Model file for the job. Use its own axes, mm. A direction names the side the tool comes from. Give positions to 0.01 mm unless a question says otherwise; leave off trailing zeros. Loops run counter-clockwise (first coordinate to the right, second up) from the corner with the lowest first, then second, coordinate; pieces in that order, holes last. Notation, with made-up numbers: (-13.75, -19) - (0.25, -19) arc R8 cw to (0.25, -11) - close; hole circle Ø7 at (88, 85). An arc over 180 degrees is marked (long way). Answer as CSV lines item,"result". Start each with the question number.
Item 1: Saw through at C-C on y = -2.75. Give the cut face in (x, z).
Item 2: Saw through at A-A on x = 0. Give the cut face in (y, z), plus the area to 3 significant figures.
Item 3: Drill centre lines: L1, parallel to Z at x = 19, y = 1.25; L2, parallel to Y at x = -2, z = 9.5; L3, parallel to X at y = 4.5, z = 10.5. Where is each one in solid material? Low to high. Write a range as from..to.
Item 4: Saw through at D-D on x = 18.5. Give the cut face in (y, z), plus the area to 3 significant figures.
Item 5: Tool access for faces 1 (the flat face through (-6, -3, 25.4)), 2 (the flat face through (18, 6.35, 6)): list every direction of +Z, -Z, +X, -X, +Y, -Y with a clear straight run to the whole face (end or side of a thin tool).
Item 6: Saw through at B-B on z = 5.5. Give the cut face in (x, y), plus the area to 3 significant figures.
Item 7: Pin check, flat tips, straight feed: pin 1 (14 mm diameter, centred on x = 19, z = 5, fed in from +Y); pin 2 (4 mm diameter, centred on y = 4.5, z = 8, fed in from +X); pin 3 (2 mm diameter, centred on x = 7, z = 14, fed in from +Y); pin 4 (2.5 mm diameter, centred on x = 16.5, y = -1.5, fed in from +Z). Stop position of each tip, or through.
Item 8: Pull direction X, two halves, no side cores. Call faces 3 (the flat face through (18, -6.35, 6)), 4 (the flat face through (25.4, 0, 3)), 5 (the cylindrical face through (-1.38, -6.2, 12.52)): pulls with the +X half, pulls with the -X half, needs draft (parallel to the pull), parting line crosses it, or undercut.
from build123d import *

# Parameters (mm, degrees)
F0_R     = 6.35
F1_DEPTH = 25.4
F0_W     = 6.35
F0_H     = 6.35
F2_DEPTH = 12.7
F3_SIZE  = 6.35


with BuildPart() as f1:
    # F0 (on Top) → F1 (new body)
    with BuildSketch(Plane.XY):
        with BuildLine():
            ThreePointArc((10.9985226281, -6.35), (12.2672579939, -3.2870018728), (12.7, 0))
            ThreePointArc((12.7, 0), (12.2672579939, 3.2870018728), (10.9985226281, 6.35))
            ThreePointArc((10.9985226281, 6.35), (-12.7, 0), (10.9985226281, -6.35))
        make_face()
        Circle(F0_R, mode=Mode.SUBTRACT)
    extrude(amount=F1_DEPTH)

    # F0 (on Top) → F2 (join)
    with BuildSketch(Plane.XY):
        with BuildLine():
            Line((19.05, 0), (12.7, 0))
            ThreePointArc((12.7, 0), (12.2672579939, -3.2870018728), (10.9985226281, -6.35))
            Line((10.9985226281, -6.35), (19.05, -6.35))
            Line((19.05, -6.35), (19.05, 0))
        make_face()
        with BuildLine():
            ThreePointArc((10.9985226281, 6.35), (12.2672579939, 3.2870018728), (12.7, 0))
            Line((12.7, 0), (19.05, 0))
            Line((19.05, 0), (19.05, 6.35))
            Line((19.05, 6.35), (10.9985226281, 6.35))
        make_face()
        with Locations((22.225, 3.175)):
            Rectangle(F0_W, F0_H)
        with Locations((22.225, -3.175)):
            Rectangle(F0_W, F0_H)
    extrude(amount=F2_DEPTH)

    # F3
    f3_edges = [f1.edges().sort_by_distance(p)[0] for p in [
        (25.4, 0, 12.7),
    ]]
    chamfer(f3_edges, length=F3_SIZE)


solid = f1.part
Responses:
1,outline,"(-12.4, 0) - (-5.72, 0) - (-5.72, 25.4) - (-12.4, 25.4) - close; (5.72, 0) - (25.4, 0) - (25.4, 6.35) - (19.05, 12.7) - (12.4, 12.7) - (12.4, 25.4) - (5.72, 25.4) - close"
2,outline,"(-12.7, 0) - (-6.35, 0) - (-6.35, 25.4) - (-12.7, 25.4) - close; (6.35, 0) - (12.7, 0) - (12.7, 25.4) - (6.35, 25.4) - close"
2,area,"323 mm2"
3,L1,"0..12.7"
3,L2,"-12.54..-6.03, 6.03..12.54"
3,L3,"-11.88..-4.48, 4.48..21.25"
4,outline,"(-6.35, 0) - (6.35, 0) - (6.35, 12.7) - (-6.35, 12.7) - close"
4,area,"161 mm2"
5,face 1,"+Z, +X, -X, +Y, -Y"
5,face 2,"+Z, -Z, +X, +Y"
6,outline,"(11, -6.35) - (25.4, -6.35) - (25.4, 6.35) - (11, 6.35) arc R12.7 ccw (long way) to start; hole circle Ø12.7 at (0, 0)"
6,area,"548 mm2"
7,pin 1,"y = 6.35"
7,pin 2,"x = 25.4"
7,pin 3,"y = 11.19"
7,pin 4,"z = 12.7"
8,face 3,"needs draft"
8,face 4,"pulls with the +X half"
8,face 5,"undercut"
